CAD build for the part. Positions are in the model's coordinates, mm. Face numbers are marked on the shaded views. A direction names the side the tool comes from. Give positions to 0.01 mm unless a question says otherwise; leave off trailing zeros. Order: outer loops, then holes, each group sorted by start corner. A loop starts at its lowest first (then second) coordinate and runs counter-clockwise, first axis right, second up.
Item 1: Which spindle directions (+Z, -Z, +X, -X, +Y, -Y) get a long thin tool onto all of the face, cutting with end or side? Do the marked faces 1, 2 and 3. Say none if no direction does.
Item 2: Flat gauge pins, fed straight in: P1, Ø6, axis at x = 19, y = -10, coming from the -Z side; P2, Ø5, axis at x = 17.5, y = -20, coming from the +Z side; P3, Ø3, axis at x = 26, z = 14, coming from the -Y side; P4, Ø6, axis at y = -8.75, z = 0, coming from the +X side. Where does each tip first touch, or does it go through?
Item 3: Wall check: L1, parallel to Y at x = 26.4, z = 13.75 (3 decimals); L2, parallel to Y at x = 11, z = 0.5; L3, parallel to Y at x = 10, z = 13. Give the ranges that are in metal, low to high.
Item 4: Two-plate mould, pull along X, no slides. Class the marked faces 4, 5 and 6: released by +X, released by -X, zero draft, split by the parting line, or undercut.
Item 5: Band-saw the part on C-C on y = -23. Give the cut face in (x, z).
Item 6: Band-saw the part on B-B on z = 0. Count the separate pieces of the cut face and the enclosed holes in it, plus the area to 3 significant figures.
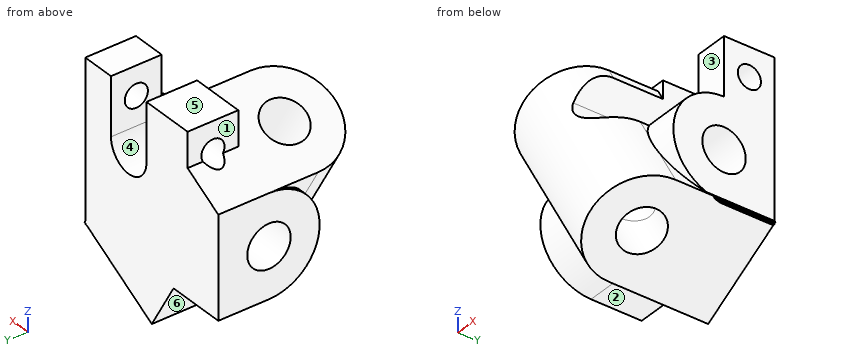
```python
from build123d import *

# Parameters (mm, degrees)
SKETCH1_R           = 3.75
BOSS_EXTRUDE1_DEPTH = 30
SKETCH2_R           = 3.75
BOSS_EXTRUDE2_DEPTH = 30
CUT_EXTRUDE1_DEPTH  = 27.0000001
SKETCH4_W           = 5.792740578
SKETCH4_H           = 10
BOSS_EXTRUDE3_DEPTH = 8.75
BOSS_EXTRUDE4_DEPTH = 8.75
SKETCH5_R           = 2
CUT_EXTRUDE2_DEPTH  = 31.0000001
SKETCH7_R           = 3.75
CUT_EXTRUDE3_DEPTH  = 31.155444666
SKETCH8_R           = 3.75
CUT_EXTRUDE4_DEPTH  = 38.57772242


with BuildPart() as part:
    # Sketch1 → Boss-Extrude1 (new body)
    with BuildSketch(Plane(origin=(0, 0, 0), x_dir=(0, 0, -1), z_dir=(1, 0, 0))):
        with BuildLine():
            Line((-8.75, 0), (8.75, 0))
            Line((8.75, 0), (8.75, 8.75))
            ThreePointArc((8.75, 8.75), (0, 17.5), (-8.75, 8.75))
            Line((-8.75, 8.75), (-8.75, 0))
        make_face()
        with Locations((0, 8.75)):
            Circle(SKETCH1_R, mode=Mode.SUBTRACT)
    extrude(amount=BOSS_EXTRUDE1_DEPTH)

    # Sketch2 → Boss-Extrude2 (add)
    with BuildSketch(Plane(origin=(-3.788861142, 0, 6.5625), x_dir=(-0.866025404, 0, -0.5), z_dir=(0.5, 0, -0.866025404))):
        with BuildLine():
            Line((-4.375, 0), (-4.375, 17.25))
            ThreePointArc((-4.375, 17.25), (-13.125, 26), (-21.875, 17.25))
            Line((-21.875, 17.25), (-21.875, 0))
            Line((-21.875, 0), (-4.375, 0))
        make_face()
        with Locations((-13.125, 17.25)):
            Circle(SKETCH2_R, mode=Mode.SUBTRACT)
    extrude(amount=BOSS_EXTRUDE2_DEPTH)

    # Sketch3 → Cut-Extrude1 (cut, through all)
    with BuildSketch(Plane.XZ):
        with BuildLine():
            Line((24.207259422, 8.75), (24.207259422, 15.67820323))
            Line((24.207259422, 15.67820323), (16.207259422, 15.67820323))
            Line((16.207259422, 15.67820323), (16.207259422, 8.75))
            ThreePointArc((16.207259422, 8.75), (20.207259422, 4.75), (24.207259422, 8.75))
        make_face()
    extrude(amount=-CUT_EXTRUDE1_DEPTH, mode=Mode.SUBTRACT)

    # Sketch4 → Boss-Extrude3 (add)
    with BuildSketch(Plane.XZ):
        with Locations((27.103629711, 13.75)):
            Rectangle(SKETCH4_W, SKETCH4_H)
    extrude(amount=-BOSS_EXTRUDE3_DEPTH)

    # Sketch6 → Boss-Extrude4 (add)
    with BuildSketch(Plane.XZ):
        Polygon((16.207259422, 15.67820323), (16.207259422, 18.75), (6.92820323, 18.75), (6.92820323, 12.75), align=None)
    extrude(amount=-BOSS_EXTRUDE4_DEPTH)

    # Sketch5 → Cut-Extrude2 (cut, through all)
    with BuildSketch(Plane(origin=(30, 0, 0), x_dir=(0, 0, -1), z_dir=(1, 0, 0))):
        with Locations(Location((-13.75, 4.375, 0), (0, 0, 60))):  # turned: the seam where the file's is
            Circle(SKETCH5_R)
    extrude(amount=-CUT_EXTRUDE2_DEPTH, mode=Mode.SUBTRACT)

    # Sketch7 → Cut-Extrude3 (cut, through all)
    with BuildSketch(Plane.ZY):
        with Locations(Location((0, 8.75, 0), (0, 0, 180))):  # turned: the seam where the file's is
            Circle(SKETCH7_R)
    extrude(amount=-CUT_EXTRUDE3_DEPTH, mode=Mode.SUBTRACT)

    # Sketch8 → Cut-Extrude4 (cut, through all)
    with BuildSketch(Plane(origin=(-3.788861142, 0, 6.5625), x_dir=(0.866025404, 0, 0.5), z_dir=(-0.5, 0, 0.866025404))):
        with Locations(Location((13.125, 17.25, 0), (0, 0, 180))):  # turned: the seam where the file's is
            Circle(SKETCH8_R)
    extrude(amount=-CUT_EXTRUDE4_DEPTH, mode=Mode.SUBTRACT)


with BuildPart() as body_2:
    # Mirror1: mirrored copy
    add(part.part.mirror(Plane(origin=(30, 0, 8.75), x_dir=(0, 0, 1), z_dir=(0, 1, 0))))


solid = body_2.part
```
The answers:
1. face 1: +Z, -X, +Y, -Y
1. face 2: -Z, -X, +Y, -Y
1. face 3: +Z, +X, -Y
2. P1: stops at z = -16.65
2. P2: stops at z = 17.11
2. P3: stops at y = -8.75
2. P4: passes through
3. L1: y = -8.75 to -6.375, -2.375 to 0
3. L2: y = -25.33 to -18.94, -15.56 to -12.47, -5.03 to 0
3. L3: y = -25.76 to -20.4, -14.1 to -6.23, -2.52 to 0
4. face 4: undercut
4. face 5: zero draft
4. face 6: released by -X
5. outline: (1.87, 9.83) - (16.87, -16.15) - (28.29, -9.56) - (20.03, 4.75) arc R4 cw to (16.21, 8.75) - (16.21, 11.37) - (13.29, 16.42) - close
6. separate pieces: 2
6. enclosed holes: 1
6. area: 383 mm2
